Part model, mm, in its own coordinate system. A direction names the side the tool comes from. Coordinates: 2 decimals unless noted, no trailing zeros. Write each loop counter-clockwise with the first axis right and the second up, starting at its lowest first coordinate (ties: lowest second). Pieces come first, ordered by that corner, then holes. Notation, with made-up numbers: (-4, 21) -> (8, 21) arc R20 ccw to (8, 45) -> close; hole circle Ø10 at (54, 64). An arc over 180 degrees is marked (long way). Write item = value, one per line. Start each with the question number.
Q1. Band-saw the part on A-A, the plane z = 13. List the corners of the cut face in (x, y).
Q2. Band-saw the part on B-B, the plane x = 27.5. List the corners of the cut face in (y, z) (3 decimals).
Q3. Pin check, flat tips, straight feed: P1, Ø5, axis at y = -35.5, z = 11, coming from the -X side; P2, Ø8, axis at y = -38, z = 6, coming from the +X side; P3, Ø12, axis at y = -11, z = 22.5, coming from the +X side; P4, Ø3, axis at y = -25, z = 4.5, coming from the +X side. Stop position of each tip, or through.
Q4. Tool access for faces 1 (the flat face through (12, 0, 16)), 2 (the flat face through (25.49, -6.26, 15.65)), 3 (the flat face through (38, -31.75, 16)): list every direction of +Z, -Z, +X, -X, +Y, -Y with a clear straight run to the whole face (end or side of a thin tool).
Q5. Band-saw the part on D-D, the plane y = -16. List the corners of the cut face in (x, z), plus the area to 3 significant figures.
Q6. Probe line 1 (Y direction, x = 29, z = 24.5); line 2 (X direction, y = -4, z = 28); line 3 (X direction, y = -11.5, z = 3). List the from-to ranges inside material, lowest first.
Q7. Band-saw the part on C-C, the plane y = -4. List the corners of the cut face in (x, z).
from build123d import *

# Parameters (mm, degrees)
F0_W      = 57.15
F0_H      = 31.75
F1_DEPTH  = 44.45
F3_DEPTH  = 12.7
F5_DEPTH  = 12.7
F7_DEPTH  = 12.7
F9_DEPTH  = 12.7
F10_DEPTH = 6.35
F11_DEPTH = 6.35
F12_DEPTH = 25.4


with BuildPart() as f1:
    # F0 (on Front) → F1 (new body)
    with BuildSketch(Plane.XZ):
        with Locations((28.575, 15.875)):
            Rectangle(F0_W, F0_H)
    extrude(amount=F1_DEPTH)

    # F2 (on Front) → F3 (cut)
    with BuildSketch(Plane.XZ):
        Polygon((19.05, 31.75), (19.05, 0), (31.75, 0), align=None)
    extrude(amount=-F3_DEPTH, mode=Mode.SUBTRACT)

    # F4 (on face) → F5 (cut)
    with BuildSketch(Plane.XZ.offset(44.45)):
        Polygon((31.75, 0), (57.15, 0), (57.15, 31.75), (19.05, 31.75), align=None)
    extrude(amount=-F5_DEPTH, mode=Mode.SUBTRACT)

    # F6 (on face) → F7 (cut)
    with BuildSketch(Plane(origin=(0, 0, 0), x_dir=(-1, 0, 0), z_dir=(0, 1, 0))):
        Polygon((-57.15, 31.75), (-57.15, 0), (-31.75, 0), (-19.05, 31.75), align=None)
    extrude(amount=-F7_DEPTH, mode=Mode.SUBTRACT)

    # F8 (on face) → F9 (cut)
    with BuildSketch(Plane.XZ.offset(31.75)):
        Polygon((44.45, 31.75), (57.15, 0), (57.15, 31.75), align=None)
    extrude(amount=-F9_DEPTH, mode=Mode.SUBTRACT)

    # F10 (add): a face of the model
    f10_faces = [f1.faces().sort_by_distance(p)[0] for p in [
        (52.9166666667, -19.05, 21.1666666667),
    ]]
    extrude(f10_faces, amount=F10_DEPTH)

    # F11 (cut): a face of the model
    f11_faces = [f1.faces().sort_by_distance(p)[0] for p in [
        (52.9166666667, -25.4, 21.1666666667),
    ]]
    extrude(f11_faces, amount=-F11_DEPTH, mode=Mode.SUBTRACT)

    # F12 (cut): a face of the model
    f12_faces = [f1.faces().sort_by_distance(p)[0] for p in [
        (52.9166666667, -19.05, 21.1666666667),
    ]]
    extrude(f12_faces, amount=-F12_DEPTH, mode=Mode.SUBTRACT)


solid = f1.part
Ans:
q1.outline = (0, -44.45) -> (26.55, -44.45) -> (26.55, -31.75) -> (51.95, -31.75) -> (51.95, -12.7) -> (26.55, -12.7) -> (26.55, 0) -> (0, 0) -> close
q2.outline = (-44.45, 0) -> (0, 0) -> (0, 10.625) -> (-12.7, 10.625) -> (-12.7, 31.75) -> (-31.75, 31.75) -> (-31.75, 10.625) -> (-44.45, 10.625) -> close
q3.P1 = 0
q3.P2 = 30.95
q3.P3 = 50.45
q3.P4 = 55.95
q4.face_1 = +Z, -Z, +X, -X, +Y
q4.face_2 = +Z, +X, +Y
q4.face_3 = +Z, +X, -Y
q5.outline = (0, 0) -> (57.15, 0) -> (44.45, 31.75) -> (0, 31.75) -> close
q5.area = 1,610 mm2
q6.line_1 = -31.75 to -12.7
q6.line_2 = 0 to 20.55
q6.line_3 = 0 to 30.55
q7.outline = (0, 0) -> (31.75, 0) -> (19.05, 31.75) -> (0, 31.75) -> close
